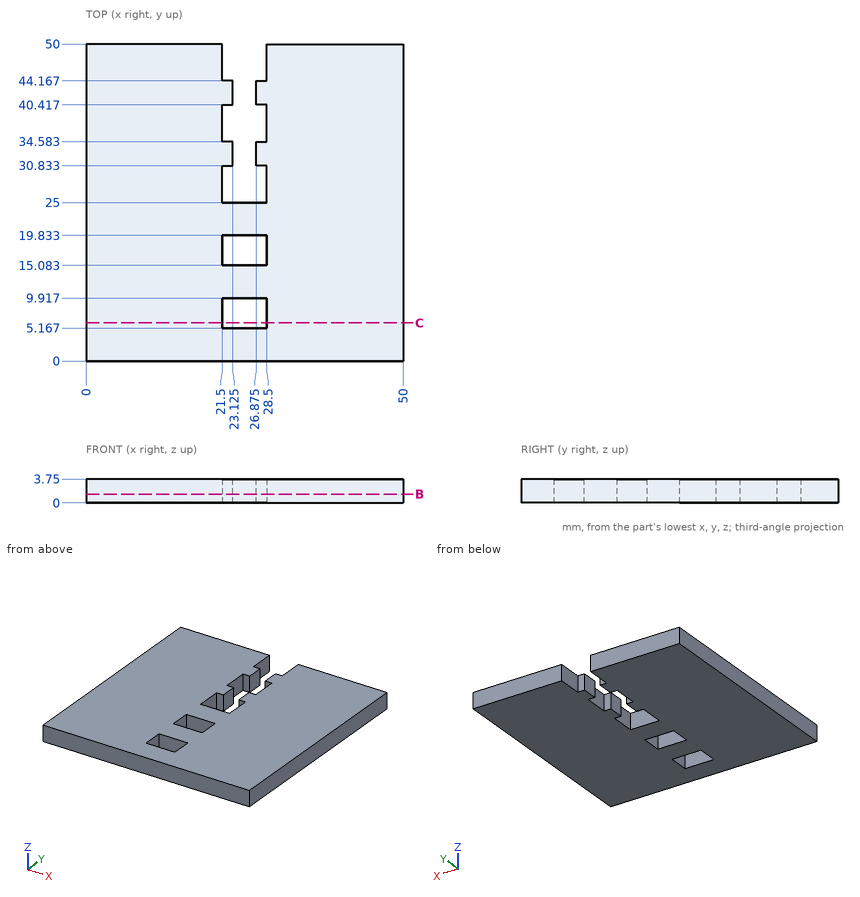
Drawing for the job (mm, zero at the part's lowest x, y, z). Coordinates: 2 decimals unless noted, no trailing zeros. Order: outer loops, then holes, each group sorted by start corner. A loop starts at its lowest first (then second) coordinate and runs counter-clockwise, first axis right, second up. Notation, with made-up numbers: (3.25, -27) -> (24.25, -27) arc R20 cw to (24.25, -14) -> close; hole circle Ø8 at (52, 42). An arc over 180 degrees is marked (long way). Return JSON: item names as keys, results as strings.
Item 1: Slice it at B-B (z = 1.35). Count the separate pieces of the cut face and the enclosed holes in it, then the cut area to 3 significant figures.
Model answer:
{"separate pieces": "1", "enclosed holes": "2", "area": "2,280 mm²"}
Item 2: Pin check, flat tips, straight feed: P1, Ø1.9, axis at y = 17, z = 2, coming from the -X side; P2, Ø0.5, axis at x = 22, z = 2, coming from the +Y side; P3, Ø1.1, axis at x = 25.5, z = 2.5, coming from the +Y side. Stop position of each tip, or through.
Model answer:
{"P1": "stops at x = 0", "P2": "stops at y = 44.17", "P3": "stops at y = 25"}
Item 3: Slice it at C-C (y = 6). Write the cut outline in (x, z).
Model answer:
{"outline": "(0, 0) -> (21.5, 0) -> (21.5, 3.75) -> (0, 3.75) -> close; (28.5, 0) -> (50, 0) -> (50, 3.75) -> (28.5, 3.75) -> close"}
Item 4: Wall check: line 1 along Y through (x, z) = (24, 0.6); line 2 along Y through (x, z) = (27, 1.35); line 3 along X through (y, z) = (39.5, 1.3). Give the ranges that are in metal, low to high. Write a range as from..to.
Model answer:
{"line 1": "y = 0..5.17, 9.92..15.08, 19.83..25", "line 2": "y = 0..5.17, 9.92..15.08, 19.83..25, 30.83..34.58, 40.42..44.17", "line 3": "x = 0..21.5, 28.5..50"}
